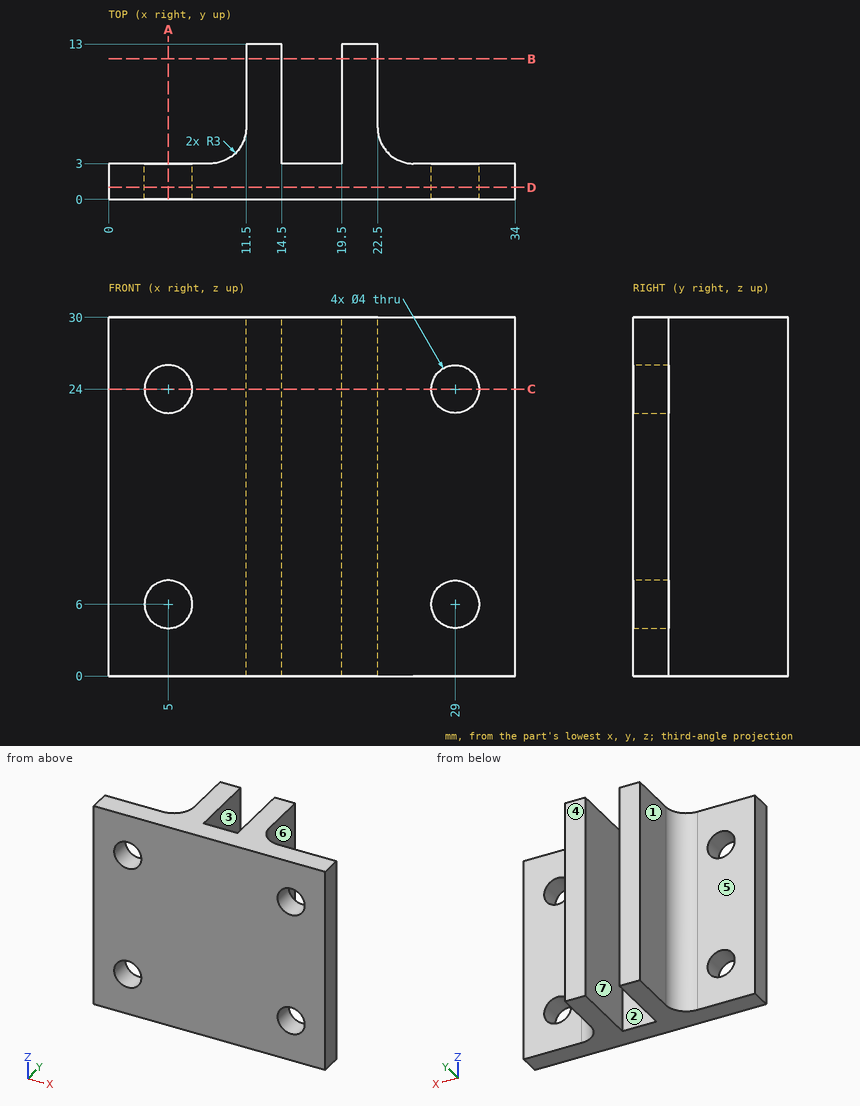
The drawing under review shows one solid part. Ordinate dimensions are in mm from its lowest x, y, z. A direction names the side the tool comes from. Round coordinates to 2 decimals unless told otherwise and drop trailing zeros. Write each loop counter-clockwise with the first axis right and the second up, starting at its lowest first coordinate (ties: lowest second). Pieces come first, ordered by that corner, then holes.
(1) Insertion check: pin 1 (3 mm diameter, centred on x = 6.5, z = 16, fed in from +Y); pin 2 (3.5 mm diameter, centred on y = 10.5, z = 10.5, fed in from +X); pin 3 (2 mm diameter, centred on y = 10.5, z = 14, fed in from -X). Each pin has a flat end and moves straight along its axis. Give the tip position at first contact, or say it passes through.
(2) We need section C-C on z = 24. Give the boundary of the cut face in (x, y).
(3) We need section D-D on y = 1. Give the boundary of the cut face in (x, z), and give its area (3 significant figures).
(4) We need section A-A on x = 5. Give the boundary of the cut face in (y, z), and give its area (3 significant figures).
(5) Machinability: for the marked faces 5, 6 and 7, which of the approach directions +Z, -Z, +X, -X, +Y, -Y give a long, thin tool a straight path to every point of the face, cutting with its end or side? Answer none if there is none.
(6) Wall thickness on L1, parallel to X at y = 2.15, z = 6; L2, parallel to Z at x = 5, y = 0.75; L3, parallel to X at y = 8, z = 24.75: over which ranges is each line inside the solid? List them lowest first.
(7) Mouldability with a two-part tool opening along X and no side actions: class the marked faces 1, 2, 3 and 4 as +X half, -X half, draft (parallel to the pull), parting line (faces both ways), or undercut.
(8) We need section B-B on y = 11.75. Give the boundary of the cut face in (x, z), and give its area (3 significant figures).
Findings below:
1. pin 1: stops at y = 3
1. pin 2: stops at x = 22.5
1. pin 3: stops at x = 11.5
2. outline: (0, 0) - (3, 0) - (3, 3) - (0, 3) - close; (7, 0) - (27, 0) - (27, 3) - (25.5, 3) arc R3 cw to (22.5, 6) - (22.5, 13) - (19.5, 13) - (19.5, 3) - (14.5, 3) - (14.5, 13) - (11.5, 13) - (11.5, 6) arc R3 cw to (8.5, 3) - (7, 3) - close; (31, 0) - (34, 0) - (34, 3) - (31, 3) - close
3. outline: (0, 0) - (34, 0) - (34, 30) - (0, 30) - close; hole circle Ø4 at (5, 6); hole circle Ø4 at (5, 24); hole circle Ø4 at (29, 6); hole circle Ø4 at (29, 24)
3. area: 970 mm2
4. outline: (0, 0) - (3, 0) - (3, 4) - (0, 4) - close; (0, 8) - (3, 8) - (3, 22) - (0, 22) - close; (0, 26) - (3, 26) - (3, 30) - (0, 30) - close
4. area: 66.0 mm2
5. face 5: +Z, -Z, -X, +Y
5. face 6: +Z, -Z, +X, +Y
5. face 7: +Z, -Z, +Y
6. L1: x = 0 to 3, 7 to 27, 31 to 34
6. L2: z = 0 to 4, 8 to 22, 26 to 30
6. L3: x = 11.5 to 14.5, 19.5 to 22.5
7. face 1: -X half
7. face 2: undercut
7. face 3: undercut
7. face 4: draft
8. outline: (11.5, 0) - (14.5, 0) - (14.5, 30) - (11.5, 30) - close; (19.5, 0) - (22.5, 0) - (22.5, 30) - (19.5, 30) - close
8. area: 180 mm2
